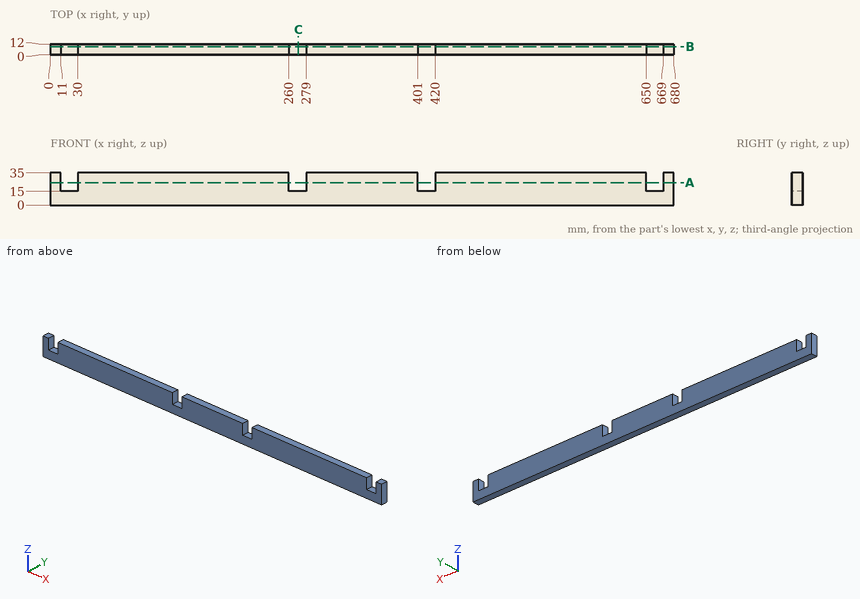
Drawing for the job (mm, zero at the part's lowest x, y, z). Coordinates: 2 decimals unless noted, no trailing zeros. Order: outer loops, then holes, each group sorted by start corner. A loop starts at its lowest first (then second) coordinate and runs counter-clockwise, first axis right, second up. Notation, with made-up numbers: (-3, -9.75) -> (44, -9.75) arc R23 ccw to (44, 16.25) -> close; hole circle Ø1 at (61, 45.25). An arc over 180 degrees is marked (long way). One line per item, written item: value.
(1) Drop a flat-ended pin along its axis: pin 1 Ø3.5 at (x, y) = (265.5, 4) entering from +Z. Give the stop position or say it passes through.
Checked values:
pin 1: z = 15
(2) Slice it at C-C, the plane x = 270.5. List the corners of the cut face in (y, z), plus the area to 3 significant figures.
Checked values:
outline: (0, 0) -> (12, 0) -> (12, 15) -> (0, 15) -> close
area: 180 mm2
(3) Probe line 1 (X direction, y = 7.75, z = 26). List the from-to ranges inside material, lowest first. Write a range as [from, to].
Checked values:
line 1: [0, 11], [30, 260], [279, 401], [420, 650], [669, 680]
(4) Slice it at B-B, the plane y = 9. List the corners of the cut face in (x, z), plus the area to 3 significant figures.
Checked values:
outline: (0, 0) -> (680, 0) -> (680, 35) -> (669, 35) -> (669, 15) -> (650, 15) -> (650, 35) -> (420, 35) -> (420, 15) -> (401, 15) -> (401, 35) -> (279, 35) -> (279, 15) -> (260, 15) -> (260, 35) -> (30, 35) -> (30, 15) -> (11, 15) -> (11, 35) -> (0, 35) -> close
area: 22,300 mm2
(5) Slice it at A-A, the plane z = 24.5. List the corners of the cut face in (x, y), plus the area to 3 significant figures.
Checked values:
outline: (0, 0) -> (11, 0) -> (11, 12) -> (0, 12) -> close; (30, 0) -> (260, 0) -> (260, 12) -> (30, 12) -> close; (279, 0) -> (401, 0) -> (401, 12) -> (279, 12) -> close; (420, 0) -> (650, 0) -> (650, 12) -> (420, 12) -> close; (669, 0) -> (680, 0) -> (680, 12) -> (669, 12) -> close
area: 7,250 mm2
